The model under review builds one solid part; all positions refer to its coordinate system, in mm. A direction names the side the tool comes from. Coordinates: 2 decimals unless noted, no trailing zeros. Write each loop counter-clockwise with the first axis right and the second up, starting at its lowest first coordinate (ties: lowest second). Pieces come first, ordered by that corner, then holes.
```python
from build123d import *

# Parameters (mm, degrees)
BOSS_EXTRUDE1_DEPTH = 2.65
CUT_EXTRUDE2_DEPTH  = 0.75
FILLET3_R           = 1.65
FILLET4_R           = 0.5


with BuildPart() as part:
    # Sketch1 → Boss-Extrude1 (new, symmetric)
    with BuildSketch(Plane(origin=(0, 0, 0), x_dir=(1, 0, 0), z_dir=(0, 1, 0))):
        with BuildLine():
            Line((-20.776037351, 4.9), (-17.775892991, 4.9))
            ThreePointArc((-17.775892991, 4.9), (-17.772061826, 5.275001496), (-17.767948266, 5.65))
            Line((-17.767948266, 5.65), (-17.017899919, 5.65))
            Line((-17.017899919, 5.65), (-17.017899919, -5.65))
            Line((-17.017899919, -5.65), (-17.767948266, -5.65))
            ThreePointArc((-17.767948266, -5.65), (-17.772061826, -5.275001496), (-17.775892991, -4.9))
            Line((-17.775892991, -4.9), (-20.776037351, -4.9))
            ThreePointArc((-20.776037351, -4.9), (-20.8, 0), (-20.776037351, 4.9))
        make_face()
    extrude(amount=BOSS_EXTRUDE1_DEPTH, both=True)

    # Sketch2 → Cut-Extrude2 (cut)
    with BuildSketch(Plane(origin=(0, 2.65, 0), x_dir=(1, 0, 0), z_dir=(0, 1, 0))):
        with BuildLine():
            Line((-17.775892991, 4.9), (-20.776037348, 4.9))
            ThreePointArc((-20.776037348, 4.9), (-20.799999997, 0), (-20.776037348, -4.9))
            Line((-20.776037348, -4.9), (-17.775892991, -4.9))
            ThreePointArc((-17.775892991, -4.9), (-17.8, 0), (-17.775892991, 4.9))
        make_face()
    cut_extrude2 = extrude(amount=-CUT_EXTRUDE2_DEPTH, mode=Mode.SUBTRACT)

    # Mirror1: Cut-Extrude2 across plane
    add(cut_extrude2.mirror(Plane.ZX), mode=Mode.SUBTRACT)

    # Fillet3
    # the kernel refuses this fillet: 1.65 mm, written as the material it takes off along each edge
    with BuildSketch(Plane(origin=(-17.017899919, 2.65, 5.65), x_dir=(0, 0, -1), z_dir=(-1, 0, 0))) as fillet3_piece_1_section:
        with BuildLine():
            CenterArc((FILLET3_R, FILLET3_R), FILLET3_R, 180, 90)
            Line((0, FILLET3_R), (-FILLET3_R * 0.02, FILLET3_R))
            Line((-FILLET3_R * 0.02, FILLET3_R), (-FILLET3_R * 0.02, -FILLET3_R * 0.02))
            Line((-FILLET3_R * 0.02, -FILLET3_R * 0.02), (FILLET3_R, -FILLET3_R * 0.02))
            Line((FILLET3_R, -FILLET3_R * 0.02), (FILLET3_R, 0))
        make_face()
    fillet3_piece_1 = extrude(amount=4.875048347, mode=Mode.PRIVATE)
    fillet3_piece_1 = fillet3_piece_1 & Plane(origin=(480.200000514, 2.277476363, -5e-09), x_dir=(-0.9999356390878598, 0, 0.011345381525254326), z_dir=(0, 1, 0)) * Cylinder(498.000000514, 17, mode=Mode.PRIVATE)
    add(fillet3_piece_1, mode=Mode.SUBTRACT)
    with BuildSketch(Plane(origin=(-21.892948266, 2.65, -5.65), x_dir=(0, -1, 0), z_dir=(1, 0, 0))) as fillet3_piece_2_section:
        with BuildLine():
            CenterArc((FILLET3_R, -FILLET3_R), FILLET3_R, 90, 90)
            Line((0, -FILLET3_R), (-FILLET3_R * 0.02, -FILLET3_R))
            Line((-FILLET3_R * 0.02, -FILLET3_R), (-FILLET3_R * 0.02, FILLET3_R * 0.02))
            Line((-FILLET3_R * 0.02, FILLET3_R * 0.02), (FILLET3_R, FILLET3_R * 0.02))
            Line((FILLET3_R, FILLET3_R * 0.02), (FILLET3_R, 0))
        make_face()
    fillet3_piece_2 = extrude(amount=4.875048347, mode=Mode.PRIVATE)
    fillet3_piece_2 = fillet3_piece_2 & Plane(origin=(480.200000325, 2.277476179, 3e-09), x_dir=(-0.9999515923510308, 0, -0.009839357430136753), z_dir=(0, 1, 0)) * Cylinder(498.000000325, 17, mode=Mode.PRIVATE)
    add(fillet3_piece_2, mode=Mode.SUBTRACT)
    with BuildSketch(Plane(origin=(-24.901037348, 1.9, 4.9), x_dir=(0, 0, -1), z_dir=(1, 0, 0))) as fillet3_piece_3_section:
        with BuildLine():
            CenterArc((FILLET3_R, -FILLET3_R), FILLET3_R, 90, 90)
            Line((0, -FILLET3_R), (-FILLET3_R * 0.02, -FILLET3_R))
            Line((-FILLET3_R * 0.02, -FILLET3_R), (-FILLET3_R * 0.02, FILLET3_R * 0.02))
            Line((-FILLET3_R * 0.02, FILLET3_R * 0.02), (FILLET3_R, FILLET3_R * 0.02))
            Line((FILLET3_R, FILLET3_R * 0.02), (FILLET3_R, 0))
        make_face()
    fillet3_piece_3 = extrude(amount=11.250144357, mode=Mode.PRIVATE)
    fillet3_piece_3 = fillet3_piece_3 & Plane(origin=(480.2, 1.526447117, 0), x_dir=(-0.9999521703614557, 0, 0.009780439121757674), z_dir=(0, 1, 0)) * Cylinder(501, 30, mode=Mode.PRIVATE)
    fillet3_piece_3 = fillet3_piece_3 - Plane(origin=(480.200000004, 1.526447117, 0), x_dir=(-0.9999515923510358, 0, 0.009839357429633357), z_dir=(0, 1, 0)) * Cylinder(498.000000004, 30, mode=Mode.PRIVATE)
    add(fillet3_piece_3, mode=Mode.SUBTRACT)
    with BuildSketch(Plane(origin=(-13.650892991, 1.9, -4.9), x_dir=(0, -1, 0), z_dir=(-1, 0, 0))) as fillet3_piece_4_section:
        with BuildLine():
            CenterArc((FILLET3_R, FILLET3_R), FILLET3_R, 180, 90)
            Line((0, FILLET3_R), (-FILLET3_R * 0.02, FILLET3_R))
            Line((-FILLET3_R * 0.02, FILLET3_R), (-FILLET3_R * 0.02, -FILLET3_R * 0.02))
            Line((-FILLET3_R * 0.02, -FILLET3_R * 0.02), (FILLET3_R, -FILLET3_R * 0.02))
            Line((FILLET3_R, -FILLET3_R * 0.02), (FILLET3_R, 0))
        make_face()
    fillet3_piece_4 = extrude(amount=11.250144357, mode=Mode.PRIVATE)
    fillet3_piece_4 = fillet3_piece_4 & Plane(origin=(480.2, 1.526445495, 0), x_dir=(-0.9999521703614557, 0, 0.009780439121757674), z_dir=(0, 1, 0)) * Cylinder(501, 30, mode=Mode.PRIVATE)
    fillet3_piece_4 = fillet3_piece_4 - Plane(origin=(480.200000325, 1.526445495, 3e-09), x_dir=(-0.9999515923510308, 0, -0.009839357430136753), z_dir=(0, 1, 0)) * Cylinder(498.000000325, 30, mode=Mode.PRIVATE)
    add(fillet3_piece_4, mode=Mode.SUBTRACT)
    with BuildSketch(Plane(origin=(-13.650892991, -1.9, -4.9), x_dir=(0, 1, 0), z_dir=(-1, 0, 0))) as fillet3_piece_5_section:
        with BuildLine():
            CenterArc((FILLET3_R, -FILLET3_R), FILLET3_R, 90, 90)
            Line((0, -FILLET3_R), (-FILLET3_R * 0.02, -FILLET3_R))
            Line((-FILLET3_R * 0.02, -FILLET3_R), (-FILLET3_R * 0.02, FILLET3_R * 0.02))
            Line((-FILLET3_R * 0.02, FILLET3_R * 0.02), (FILLET3_R, FILLET3_R * 0.02))
            Line((FILLET3_R, FILLET3_R * 0.02), (FILLET3_R, 0))
        make_face()
    fillet3_piece_5 = extrude(amount=11.250144357, mode=Mode.PRIVATE)
    fillet3_piece_5 = fillet3_piece_5 & Plane(origin=(480.2, -1.526445495, 0), x_dir=(-0.9999521703614557, 0, 0.009780439121757674), z_dir=(0, 1, 0)) * Cylinder(501, 30, mode=Mode.PRIVATE)
    fillet3_piece_5 = fillet3_piece_5 - Plane(origin=(480.200000325, -1.526445495, 3e-09), x_dir=(-0.9999515923510308, 0, -0.009839357430136753), z_dir=(0, 1, 0)) * Cylinder(498.000000325, 30, mode=Mode.PRIVATE)
    add(fillet3_piece_5, mode=Mode.SUBTRACT)
    with BuildSketch(Plane(origin=(-24.901037348, -1.9, 4.9), x_dir=(0, 0, -1), z_dir=(1, 0, 0))) as fillet3_piece_6_section:
        with BuildLine():
            CenterArc((FILLET3_R, FILLET3_R), FILLET3_R, 180, 90)
            Line((0, FILLET3_R), (-FILLET3_R * 0.02, FILLET3_R))
            Line((-FILLET3_R * 0.02, FILLET3_R), (-FILLET3_R * 0.02, -FILLET3_R * 0.02))
            Line((-FILLET3_R * 0.02, -FILLET3_R * 0.02), (FILLET3_R, -FILLET3_R * 0.02))
            Line((FILLET3_R, -FILLET3_R * 0.02), (FILLET3_R, 0))
        make_face()
    fillet3_piece_6 = extrude(amount=11.250144357, mode=Mode.PRIVATE)
    fillet3_piece_6 = fillet3_piece_6 & Plane(origin=(480.2, -1.526447117, 0), x_dir=(-0.9999521703614557, 0, 0.009780439121757674), z_dir=(0, 1, 0)) * Cylinder(501, 30, mode=Mode.PRIVATE)
    fillet3_piece_6 = fillet3_piece_6 - Plane(origin=(480.200000004, -1.526447117, 0), x_dir=(-0.9999515923510358, 0, 0.009839357429633357), z_dir=(0, -1, 0)) * Cylinder(498.000000004, 30, mode=Mode.PRIVATE)
    add(fillet3_piece_6, mode=Mode.SUBTRACT)
    with BuildSketch(Plane(origin=(-21.892948266, -2.65, -5.65), x_dir=(0, 0, 1), z_dir=(1, 0, 0))) as fillet3_piece_7_section:
        with BuildLine():
            CenterArc((FILLET3_R, -FILLET3_R), FILLET3_R, 90, 90)
            Line((0, -FILLET3_R), (-FILLET3_R * 0.02, -FILLET3_R))
            Line((-FILLET3_R * 0.02, -FILLET3_R), (-FILLET3_R * 0.02, FILLET3_R * 0.02))
            Line((-FILLET3_R * 0.02, FILLET3_R * 0.02), (FILLET3_R, FILLET3_R * 0.02))
            Line((FILLET3_R, FILLET3_R * 0.02), (FILLET3_R, 0))
        make_face()
    fillet3_piece_7 = extrude(amount=4.875048347, mode=Mode.PRIVATE)
    fillet3_piece_7 = fillet3_piece_7 & Plane(origin=(480.200000325, -2.27747614, 3e-09), x_dir=(-0.9999515923510308, 0, -0.009839357430136753), z_dir=(0, 1, 0)) * Cylinder(498.000000325, 17, mode=Mode.PRIVATE)
    add(fillet3_piece_7, mode=Mode.SUBTRACT)
    with BuildSketch(Plane(origin=(-17.017899919, -2.65, 5.65), x_dir=(0, 0, -1), z_dir=(-1, 0, 0))) as fillet3_piece_8_section:
        with BuildLine():
            CenterArc((FILLET3_R, -FILLET3_R), FILLET3_R, 90, 90)
            Line((0, -FILLET3_R), (-FILLET3_R * 0.02, -FILLET3_R))
            Line((-FILLET3_R * 0.02, -FILLET3_R), (-FILLET3_R * 0.02, FILLET3_R * 0.02))
            Line((-FILLET3_R * 0.02, FILLET3_R * 0.02), (FILLET3_R, FILLET3_R * 0.02))
            Line((FILLET3_R, FILLET3_R * 0.02), (FILLET3_R, 0))
        make_face()
    fillet3_piece_8 = extrude(amount=4.875048347, mode=Mode.PRIVATE)
    fillet3_piece_8 = fillet3_piece_8 & Plane(origin=(480.200000514, -2.277476363, -5e-09), x_dir=(-0.9999356390878598, 0, 0.011345381525254326), z_dir=(0, 1, 0)) * Cylinder(498.000000514, 17, mode=Mode.PRIVATE)
    add(fillet3_piece_8, mode=Mode.SUBTRACT)

    # Fillet4
    fillet4_edges = [part.edges().sort_by_distance(p)[0] for p in [
        (-20.776037351, 0, 4.9),
        (-20.799999997, -1.9, 0),
        (-20.799999997, 1.9, 0),
        (-20.776037351, 0, -4.9),
        (-20.780531146, -1.416733553, -4.416718844),
        (-20.780531153, 1.416733542, -4.416718836),
        (-20.780531153, 1.416733544, 4.416718836),
        (-20.780531146, -1.416733553, 4.416718845),
    ]]
    fillet(fillet4_edges, radius=FILLET4_R)


solid = part.part
```
Item 1: Take a section at B-B, the plane y = 2.2. Write out the cut boundary in (x, z).
Solved:
outline: (-17.78, -4.9) arc R498 ccw to (-17.77, -5.13) - (-17.02, -5.13) - (-17.02, 5.13) - (-17.77, 5.13) arc R498 ccw to (-17.78, 4.9) arc R498 ccw to start
Item 2: Take a section at A-A, the plane x = -19.7. Write out the cut boundary in (y, z), plus the area to 3 significant figures.
Solved:
outline: (-1.9, -3.25) arc R1.65 ccw to (-0.25, -4.9) - (0.25, -4.9) arc R1.65 ccw to (1.9, -3.25) - (1.9, 3.25) arc R1.65 ccw to (0.25, 4.9) - (-0.25, 4.9) arc R1.65 ccw to (-1.9, 3.25) - close
area: 34.9 mm2
Item 3: Machinability: for faces 1 (the face through (-19.05, 1.429, 4.404)), 2 (the face through (-19.05, -1.404, 4.429)), 3 (the face through (-19, -1.9, 0)), 4 (the face through (-19.015, 1.429, -4.404)), which of the approach directions +Z, -Z, +X, -X, +Y, -Y give a long, thin tool a straight path to every point of the face, cutting with its end or side? Answer none if there is none.
Solved:
face 1: +Z, -X, +Y
face 2: +Z, -X, -Y
face 3: +Z, -Z, -X, -Y
face 4: -Z, -X, +Y
Item 4: For pin 1 (1.5 mm diameter, centred on x = -19, y = 1, fed in from -Z); pin 2 (1.3 mm diameter, centred on x = -19.5, z = 1, fed in from +Y); pin 3 (1.3 mm diameter, centred on x = -19.5, z = 1, fed in from -Y), all flat-tipped, find the tip position at first contact; note any pin that passes through.
Solved:
pin 1: stops at z = -4.9
pin 2: stops at y = 1.9
pin 3: stops at y = -1.9
Item 5: Take a section at C-C, the plane y = -2.05. Write out the cut boundary in (x, z), plus the area to 3 significant figures.
Solved:
outline: (-17.78, -4.9) arc R498 ccw to (-17.77, -5.27) - (-17.02, -5.27) - (-17.02, 5.27) - (-17.77, 5.27) arc R498 ccw to (-17.78, 4.9) arc R498 ccw to start
area: 8.15 mm2
Item 6: To check wall thickness, follow line 1 along Y through (x, z) = (-18.3, 3); line 2 along Z through (x, y) = (-19, 0.35); line 3 along X through (y, z) = (1.9, -4.75). State the ranges of each line that lie inside material, in increasing order.
Solved:
line 1: y = -1.9 to 1.9
line 2: z = -4.9 to 4.9
line 3: x = -17.78 to -17.02
